from build123d import *

# Parameters (mm, degrees)
F0_R     = 19.05
F1_DEPTH = 17.78
F4_R     = 11.5415113059
F3_R     = 20.1893668286
F6_T     = -2.54


with BuildPart() as f1:
    # F0 (on Top) → F1 (new body)
    with BuildSketch(Plane.XY):
        Circle(F0_R)
    extrude(amount=F1_DEPTH)

    # F4 (on face) → F5 section 0
    with BuildSketch(Plane.XY.offset(17.78)):
        Circle(F4_R)
    # F3 (on offset) → F5 section 1
    with BuildSketch(Plane.XY.offset(55.88)):
        Circle(F3_R)
    loft()

    # F6
    f6_openings = [f1.faces().sort_by_distance(p)[0] for p in [
        (0, 0, 0),
        (0, 0, 55.88),
    ]]
    offset(amount=F6_T, openings=f6_openings, kind=Kind.INTERSECTION)


solid = f1.part
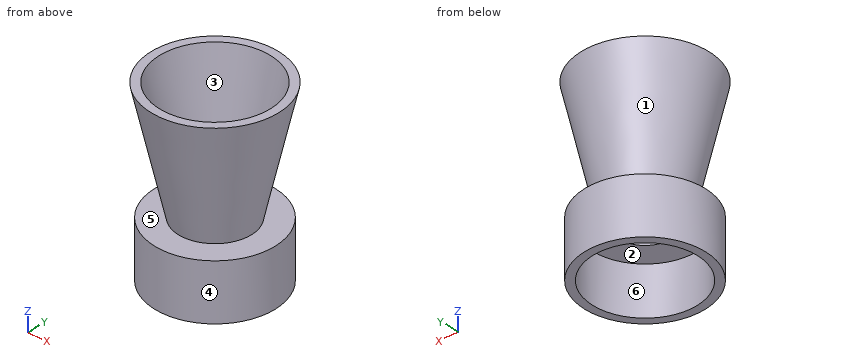
Verification items for the finished model (mm, model axes). Face numbers are marked on the shaded views. A direction names the side the tool comes from. Coordinates: 2 decimals unless noted, no trailing zeros. Write each loop counter-clockwise with the first axis right and the second up, starting at its lowest first coordinate (ties: lowest second). Pieces come first, ordered by that corner, then holes. Notation, with made-up numbers: (1.5, 44.5) -> (56.5, 44.5) arc R32 ccw to (56.5, 77.5) -> close; hole circle Ø11 at (77, -30.75). An arc over 180 degrees is marked (long way). One line per item, written item: value. Start each with the question number.
Q1. Cross-section at C-C on z = 21. Enter the section's corners in (x, y), and give its area (3 significant figures).
Q2. Cross-section at B-B on z = 12. Enter the section's corners in (x, y), and give its area (3 significant figures).
Q3. Cross-section at A-A on x = 0. Enter the section's corners in (y, z), and give its area (3 significant figures).
Q4. Mould release check, pull along Y, two halves, no side actions. Record for the marked faces 4, 5 and 6: pulls with the +Y half, pulls with the -Y half, needs draft (parallel to the pull), parting line crosses it, or undercut.
Q5. Access from +Z, -Z, +X, -X, +Y, -Y to the whole of each face (thin tool, end or side, straight path). Record for the marked faces 1, 2 and 3.
Q6. Go/stop test with flat-tipped pins: P1, Ø3, axis at x = -4.5, z = 47.5, coming from the -Y side; P2, Ø12, axis at y = -9, z = 26.5, coming from the -X side; P3, Ø2, axis at x = -13, y = -4.5, coming from the -Z side. Record where each tip stops, or that it passes through.
Q7. Thickness scan on L1, parallel to Y at x = 0, z = 8.5; L2, parallel to Y at x = 10, z = 31; L3, parallel to X at y = -1.5, z = 49.5. Record the ranges inside material, lowest first. Write a range as from..to.
Checked values:
1. outline: circle Ø24.54 at (0, 0); hole circle Ø19.34 at (0, 0)
1. area: 180 mm²
2. outline: circle Ø38.1 at (0, 0); hole circle Ø33.02 at (0, 0)
2. area: 284 mm²
3. outline: (-20.19, 55.88) -> (-11.54, 17.78) -> (-19.05, 17.78) -> (-19.05, 0) -> (-16.51, 0) -> (-16.51, 15.24) -> (-8.36, 15.24) -> (-17.58, 55.88) -> close; (8.36, 15.24) -> (16.51, 15.24) -> (16.51, 0) -> (19.05, 0) -> (19.05, 17.78) -> (11.54, 17.78) -> (20.19, 55.88) -> (17.58, 55.88) -> close
3. area: 329 mm²
4. face 4: parting line crosses it
4. face 5: needs draft
4. face 6: undercut
5. face 1: none
5. face 2: -Z
5. face 3: +Z
6. P1: stops at y = -18.21
6. P2: stops at x = -13.71
6. P3: stops at z = 15.24
7. L1: y = -19.05..-16.51, 16.51..19.05
7. L2: y = -10.56..-6.52, 6.52..10.56
7. L3: x = -18.68..-16.07, 16.07..18.68
